Verification items for the finished model (mm, model axes). A direction names the side the tool comes from. Give positions to 0.01 mm unless a question says otherwise; leave off trailing zeros. Loops run counter-clockwise (first coordinate to the right, second up) from the corner with the lowest first, then second, coordinate; pieces in that order, holes last. Notation, with made-up numbers: M 45.25,58 L 57.25,58 A5 cw 57.25,65 Z; hole C 88,-20 d3. An arc over 180 degrees is marked long. Use CSV: the item, a comma, the result in double quotes.
from build123d import *

# Parameters (mm, degrees)
SKETCH1_W      = 15
SKETCH1_H      = 5
EXTRUDE1_DEPTH = 3.175


with BuildPart() as part:
    # Sketch1 → Extrude1 (new body)
    with BuildSketch(Plane.XY):
        Polygon((92.127144536, 5.990828295), (92.127144536, 12.990828295), (85.777144536, 12.990828295), (85.777144536, 20.540828295), (76.937144536, 20.540828295), (76.937144536, 19.290828295), (74.687144536, 19.290828295), (74.687144536, 20.540828295), (71.027144536, 20.540828295), (71.027144536, 23.440828295), (74.687144536, 23.440828295), (74.687144536, 24.690828295), (76.937144536, 24.690828295), (76.937144536, 23.440828295), (85.777144536, 23.440828295), (85.777144536, 30.990828295), (92.127144536, 30.990828295), (92.127144536, 37.990828295), (-12.872855464, 37.990828295), (-12.872855464, 30.990828295), (-6.522855464, 30.990828295), (-6.522855464, 23.440828295), (2.317144536, 23.440828295), (2.317144536, 24.690828295), (4.567144536, 24.690828295), (4.567144536, 23.440828295), (8.227144536, 23.440828295), (8.227144536, 20.540828295), (4.567144536, 20.540828295), (4.567144536, 19.290828295), (2.317144536, 19.290828295), (2.317144536, 20.540828295), (-6.522855464, 20.540828295), (-6.522855464, 12.990828295), (-12.872855464, 12.990828295), (-12.872855464, 5.990828295), align=None)
        with Locations((9.627144536, 13.490828295)):
            Rectangle(SKETCH1_W, SKETCH1_H, mode=Mode.SUBTRACT)
        with Locations((69.627144536, 13.490828295)):
            Rectangle(SKETCH1_W, SKETCH1_H, mode=Mode.SUBTRACT)
    extrude(amount=EXTRUDE1_DEPTH)


solid = part.part
(1) Tool access check on faces 5 (the flat face through (3, 19.291, 2)), 6 (the flat face through (85.777, 17, 2)), 7 (the flat face through (-2, 20.541, 2)). Record the directions out of +Z, -Z, +X, -X, +Y, -Y that give a thin tool (end or side, any length) a straight path to the whole face; none if there is none.
Calculated:
face 5,"+Z, -Z"
face 6,"+Z, -Z, +X"
face 7,"+Z, -Z, -X"
(2) Section check C-C on y = 28.5. Record the cut outline in (x, z) (3 decimals).
Calculated:
outline,"M -6.523,0 L 85.777,0 L 85.777,3.175 L -6.523,3.175 Z"
(3) Depth check by flat-ended pin: pin 1 Ø0.6 at (y, z) = (20, 1.5) entering from -X; pin 2 Ø0.9 at (y, z) = (22.5, 1) entering from +X; pin 3 Ø1 at (y, z) = (24.5, 1) entering from +X. Enter the tip coordinate at first touch or a pass-through.
Calculated:
pin 1,"stops at x = -6.52"
pin 2,"stops at x = 71.03"
pin 3,"stops at x = 85.78"
(4) Section check D-D on z = 2.25. Count the separate pieces of the cut face and the enclosed holes in it, plus the area to 3 significant figures.
Calculated:
separate pieces,"1"
enclosed holes,"2"
area,"2,880 mm²"
(5) Section check B-B on y = 14. Record the cut outline in (x, z) (3 decimals).
Calculated:
outline,"M -6.523,0 L 2.127,0 L 2.127,3.175 L -6.523,3.175 Z; M 17.127,0 L 62.127,0 L 62.127,3.175 L 17.127,3.175 Z; M 77.127,0 L 85.777,0 L 85.777,3.175 L 77.127,3.175 Z"
(6) Scan lines: L1, parallel to X at y = 12, z = 2.75; L2, parallel to X at y = 13.5, z = 1.4; L3, parallel to Y at x = 79.5, z = 2.7. Record each from-to range of solid material in increasing order. Write a range as from..to.
Calculated:
L1,"x = -12.87..2.13, 17.13..62.13, 77.13..92.13"
L2,"x = -6.52..2.13, 17.13..62.13, 77.13..85.78"
L3,"y = 5.99..20.54, 23.44..37.99"
(7) Section check A-A on x = 67. Record the cut outline in (y, z) (3 decimals), plus the area to 3 significant figures.
Calculated:
outline,"M 5.991,0 L 10.991,0 L 10.991,3.175 L 5.991,3.175 Z; M 15.991,0 L 37.991,0 L 37.991,3.175 L 15.991,3.175 Z"
area,"85.7 mm²"
(8) Mould release check, pull along X, two halves, no side actions. Record for faces 1 (the flat face through (71.027, 22, 2)), 2 (the flat face through (-12.873, 10, 2)), 3 (the flat face through (39, 22, 0)), 4 (the flat face through (10, 15.991, 2)): released by +X, released by -X, zero draft, split by the parting line, or undercut.
Calculated:
face 1,"released by +X"
face 2,"released by -X"
face 3,"zero draft"
face 4,"undercut"
